from build123d import *

# Parameters (mm, degrees)
F0_W     = 44.45
F0_H     = 31.75
F1_DEPTH = 19.05
F2_W     = 19.05
F2_H     = 10.2438246012
F3_DEPTH = 25.4
F4_W     = 31.75
F4_H     = 12.7
F5_DEPTH = 50.8
F7_W     = 12.7
F7_H     = 31.75
F8_DEPTH = 25.4
F6_W     = 12.7
F6_H     = 12.7
F9_DEPTH = 25.4


with BuildPart() as f1:
    # F0 (on Front) → F1 (new body)
    with BuildSketch(Plane.XZ):
        with Locations((-22.225, 15.875)):
            Rectangle(F0_W, F0_H)
    extrude(amount=F1_DEPTH)

    # F2 (on face) → F3 (cut)
    with BuildSketch(Plane.XZ.offset(19.05)):
        with Locations((-22.225, 26.6280876994)):
            Rectangle(F2_W, F2_H)
    extrude(amount=-F3_DEPTH, mode=Mode.SUBTRACT)

    # F4 (on face) → F5 (join)
    with BuildSketch(Plane.XZ.offset(19.05)):
        with Locations((-15.875, 6.35)):
            Rectangle(F4_W, F4_H)
    extrude(amount=F5_DEPTH)

    # F7 (on face) → F8 (cut)
    with BuildSketch(Plane.XY.offset(12.7)):
        with Locations((-15.875, -53.975)):
            Rectangle(F7_W, F7_H)
    extrude(amount=-F8_DEPTH, mode=Mode.SUBTRACT)

    # F6 (on face) → F9 (cut)
    with BuildSketch(Plane.XZ.offset(69.85)):
        with Locations((-15.875, 6.35)):
            Rectangle(F6_W, F6_H)
    extrude(amount=-F9_DEPTH, mode=Mode.SUBTRACT)


solid = f1.part
The listing builds one solid part. Answer for the finished solid, in the listing's coordinates (mm). A direction names the side the tool comes from. Give positions to 0.01 mm unless a question says otherwise; leave off trailing zeros. Write each loop counter-clockwise with the first axis right and the second up, starting at its lowest first coordinate (ties: lowest second). Pieces come first, ordered by that corner, then holes.
1) Find the intervals of material crossed by L1, parallel to X at y = -5, z = 25; L2, parallel to Z at x = -17, y = -22.5; L3, parallel to Y at x = -12.5, z = 21, in increasing order.
2) Given P1, Ø9.5, axis at x = -20, y = -32.5, coming from the +Z side; P2, Ø1, axis at x = -12, y = -58, coming from the +Z side; P3, Ø4, axis at x = -31.5, y = -23, coming from the -Z side; P4, Ø9.5, axis at x = -23, y = -11.5, coming from the +Z side, each flat-ended and moving along its own axis, determine where each tip first touches the part or whether it passes through.
3) Section D-D (z = 10.5) is taken. Write down the section's boundary in (x, y) (3 decimals).
4) For a pull along X with two mould halves and no side action, classify faces 1 (the face through (0, -27, 12)), 2 (the face through (-9.525, -54, 6)), 3 (the face through (-38, -9, 31.75)), 4 (the face through (-31.75, -44, 6)) as pulls with the +X half, pulls with the -X half, needs draft (parallel to the pull), parting line crosses it, or undercut.
5) A tool of negligible diameter and unlimited length cuts with its end or side. For faces 5 (the face through (-44.45, -9, 16)), 6 (the face through (-16, -38.1, 6)), 7 (the face through (-22, -10, 21.506)), 8 (the face through (-23, -44, 12.7)), from which of +Z, -Z, +X, -X, +Y, -Y can it reach the whole face along a straight path? Write none if from no direction.
6) Section B-B (y = -56) is taken. Write down the section's boundary in (x, z) (3 decimals).
7) Section A-A (z = 28) is taken. Write down the section's boundary in (x, y), and give its area (3 significant figures).
8) Section C-C (y = -13) is taken. Write down the section's boundary in (x, z), and give its area (3 significant figures).
Response:
1. L1: x = -44.45 to -31.75, -12.7 to 0
1. L2: z = 0 to 12.7
1. L3: y = -19.05 to 0
2. P1: stops at z = 12.7
2. P2: passes through
2. P3: stops at z = 0
2. P4: stops at z = 21.51
3. outline: (-44.45, -19.05) - (-31.75, -19.05) - (-31.75, -69.85) - (-22.225, -69.85) - (-22.225, -38.1) - (-9.525, -38.1) - (-9.525, -69.85) - (0, -69.85) - (0, 0) - (-44.45, 0) - close
4. face 1: pulls with the +X half
4. face 2: undercut
4. face 3: needs draft
4. face 4: pulls with the -X half
5. face 5: +Z, -Z, -X, +Y, -Y
5. face 6: +Z, -Z, -Y
5. face 7: +Z, +Y, -Y
5. face 8: +Z, +X, -X, -Y
6. outline: (-31.75, 0) - (-22.225, 0) - (-22.225, 12.7) - (-31.75, 12.7) - close; (-9.525, 0) - (0, 0) - (0, 12.7) - (-9.525, 12.7) - close
7. outline: (-44.45, -19.05) - (-31.75, -19.05) - (-31.75, 0) - (-44.45, 0) - close; (-12.7, -19.05) - (0, -19.05) - (0, 0) - (-12.7, 0) - close
7. area: 484 mm2
8. outline: (-44.45, 0) - (0, 0) - (0, 31.75) - (-12.7, 31.75) - (-12.7, 21.51) - (-31.75, 21.51) - (-31.75, 31.75) - (-44.45, 31.75) - close
8. area: 1,220 mm2
